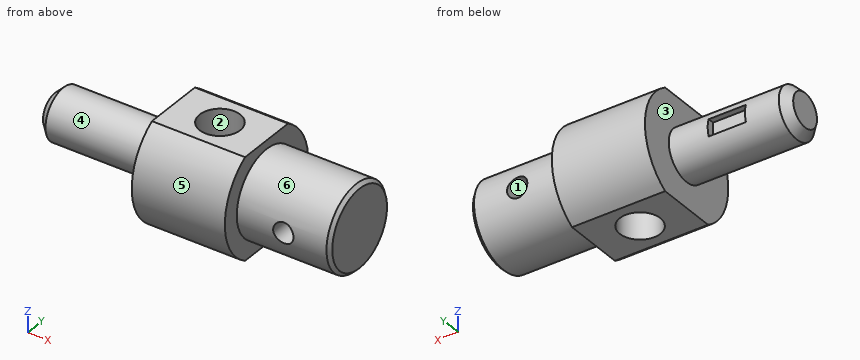
from build123d import *

# Parameters (mm, degrees)
CUT_EXTRUDE_1_DEPTH      = 135.443296597
SKETCH_3_W               = 22
SKETCH_3_H               = 4.5
CUT_EXTRUDE_2_DEPTH      = 5
HOLE_WIZARD_24_0_24_1_D  = 24
CUT_EXTRUDE_3_DEPTH      = 186.809041761
CUT_EXTRUDE_3_DEPTH_BACK = 186.809041761
SKETCH_8_R               = 6
CHAMFER_1_SIZE           = 2
CHAMFER_2_SIZE           = 5


with BuildPart() as part:
    # Эскиз1 → Повернуть1 (revolve)
    with BuildSketch(Plane.XY, mode=Mode.PRIVATE) as revolve_1_sk:
        Polygon((0, 0), (0, 15), (70, 15), (70, 35), (125, 35), (125, 25), (180, 25), (180, 0), align=None)
    revolve(revolve_1_sk.sketch.rotate(Axis((0, 0, 0), (-1, 0, 0)), 90), axis=Axis((0, 0, 0), (-1, 0, 0)))

    # Эскиз2 → Вырез-Вытянуть1 (cut, symmetric)
    with BuildSketch(Plane(origin=(125, 0, 0), x_dir=(0, 0, -1), z_dir=(1, 0, 0))):
        Polygon((-30, 195.8007333), (-30, 18.027756377), (-30, -18.027756377), (-30, -195.8007333), (-385.545953846, -195.8007333), (-385.545953846, 195.8007333), align=None)
    cut_extrude_1 = extrude(amount=CUT_EXTRUDE_1_DEPTH, both=True, mode=Mode.SUBTRACT)

    # Зеркальное отражение1: Вырез-Вытянуть1 across plane
    add(cut_extrude_1.mirror(Plane.XY), mode=Mode.SUBTRACT)

    # Эскиз3 → Вырез-Вытянуть2 (cut, symmetric)
    with BuildSketch(Plane.XY):
        with Locations((36, 12.75)):
            Rectangle(SKETCH_3_W, SKETCH_3_H)
    extrude(amount=CUT_EXTRUDE_2_DEPTH, both=True, mode=Mode.SUBTRACT)

    # Диаметр отверстия Ø24.0 (24)1 (through all)
    with Locations(Plane.XY.offset(30)):
        with Locations((97.5, 0)):
            Hole(HOLE_WIZARD_24_0_24_1_D / 2)

    # Эскиз8 → Вырез-Вытянуть3 (cut, two sides: drawn at the far end of the back side and taken through both)
    with BuildSketch(Plane(origin=(0, 0, 0), x_dir=(1, 0, 0), z_dir=(0, 1, 0)).offset(-CUT_EXTRUDE_3_DEPTH_BACK)):
        with Locations(Location((152.5, 0, 0), (0, 0, 270))):
            Circle(SKETCH_8_R)
    extrude(amount=CUT_EXTRUDE_3_DEPTH + CUT_EXTRUDE_3_DEPTH_BACK, mode=Mode.SUBTRACT)

    # Фаска1
    chamfer_1_edges = [part.edges().sort_by_distance(p)[0] for p in [
        (180, 0, 25),
    ]]
    chamfer(chamfer_1_edges, length=CHAMFER_1_SIZE)

    # Фаска2
    chamfer_2_edges = [part.edges().sort_by_distance(p)[0] for p in [
        (0, 0, 15),
    ]]
    chamfer(chamfer_2_edges, length=CHAMFER_2_SIZE)


solid = part.part
Input: part model. Units: mm. Frame: model coordinates. Face numbers are marked on the shaded views. A direction names the side the tool comes from. Coordinates: 2 decimals unless noted, no trailing zeros. Order: outer loops, then holes, each group sorted by start corner. A loop starts at its lowest first (then second) coordinate and runs counter-clockwise, first axis right, second up. Notation, with made-up numbers: M -25.75,18.5 L 26.25,18.5 A35 cw 26.25,57.5 Z; hole C 52.25,67.5 d11. An arc over 180 degrees is marked long. Answer as CSV lines item,"result".
1. Section B-B (x = 97.5). Return the cut outline in (y, z), then the cut area to 3 significant figures.
Reported:
outline,"M -18.03,-30 L -12,-30 L -12,30 L -18.03,30 A35 ccw Z; M 12,-30 L 18.03,-30 A35 ccw 18.03,30 L 12,30 Z"
area,"2,160 mm2"
2. First-contact query: P1, Ø5, axis at x = 159.5, y = -2, coming from the +Z side; P2, Ø1.5, axis at x = 161.5, z = 7, coming from the +Y side; P3, Ø8, axis at y = 6.5, z = -18.5, coming from the -X side. Flat tips, straight axial feed; report the tip coordinate or a pass-through.
Reported:
P1,"z = 25"
P2,"y = 24.21"
P3,"x = 70"
3. Material intervals for line 1 (Y direction, x = 97.5, z = -1); line 2 (Z direction, x = 126.5, y = 0.5) (3 decimals); line 3 (X direction, y = 8, z = 18), sorted ascending. Write a range as from..to.
Reported:
line 1,"-34.99..-12, 12..34.99"
line 2,"-24.995..24.995"
line 3,"70..88.56, 106.44..180"
4. Section A-A (y = 0). Return the cut outline in (x, z).
Reported:
outline,"M 0,-10 L 5,-15 L 70,-15 L 70,-30 L 85.5,-30 L 85.5,30 L 70,30 L 70,15 L 5,15 L 0,10 Z; M 109.5,-30 L 125,-30 L 125,-25 L 178,-25 L 180,-23 L 180,23 L 178,25 L 125,25 L 125,30 L 109.5,30 Z; hole C 152.5,0 d12"
5. Section C-C (z = 0). Return the cut outline in (x, y).
Reported:
outline,"M 0,-10 L 5,-15 L 70,-15 L 70,-35 L 125,-35 L 125,-25 L 146.5,-25 L 146.5,25 L 125,25 L 125,35 L 70,35 L 70,15 L 47,15 L 47,10.5 L 25,10.5 L 25,15 L 5,15 L 0,10 Z; M 158.5,-25 L 178,-25 L 180,-23 L 180,23 L 178,25 L 158.5,25 Z; hole C 97.5,0 d24"
6. Section D-D (x = 130.5). Return the cut outline in (y, z).
Reported:
outline,"C 0,0 d50"
7. Access query for the marked faces 5 and 6. Directions: +Z, -Z, +X, -X, +Y, -Y. A direction counts if a zero-diameter tool reaches every point of the face in a straight line with its end or side. Return the directions, or none.
Reported:
face 5,"+X, -X, -Y"
face 6,"+X"
8. Pull-direction query (X, two-part tool) for the marked faces 1, 2, 3 and 4; classes: released by +X, released by -X, zero draft, split by the parting line, or undercut.
Reported:
face 1,"undercut"
face 2,"undercut"
face 3,"released by -X"
face 4,"zero draft"
